```python
from build123d import *

# Parameters (mm, degrees)
F1_DEPTH     = 12
F2_T1_DEPTH  = 40.9442549995
F2_T3_DEPTH  = 65.4442549995
F2_T5_DEPTH  = 40.9442549995
F2_T7_DEPTH  = 10.4442549995
F2_T9_DEPTH  = 10.4442549995
F2_T12_ANGLE = 68.042658845
F3_W         = 6
F3_H         = 5
F4_DEPTH     = 50.251
F8_DEPTH     = 70.251
F10_DEPTH    = 3


# Not quite as in the source:
# - a fillet or chamfer that OpenCascade refuses, or shapes differently, is made with other operations: its cross-section is extruded or revolved along the edge and cut away or added


with BuildPart() as f1:
    # F0 (on Top) → F1 (new body)
    with BuildSketch(Plane.XY):
        with BuildLine():
            Line((-35.125, 35.3986228546), (-30.125, 0))
            Line((-30.125, 0), (0, 0))
            Line((0, 0), (0, 1.25))
            Line((0, 1.25), (-29.0391526732, 1.25))
            Line((-29.0391526732, 1.25), (-33.8579983297, 35.3660999978))
            Line((-33.8579983297, 35.3660999978), (-33.0027387168, 39.7740071493))
            ThreePointArc((-33.0027387168, 39.7740071493), (-17.1340283274, 46.6501181236), (0, 49))
            Line((0, 49), (0, 50.25))
            ThreePointArc((0, 50.25), (-17.738073715, 47.7785625378), (-34.125, 40.5525048866))
            Line((-34.125, 40.5525048866), (-35.125, 35.3986228546))
        make_face()
        with BuildLine():
            Line((0, 1.25), (0, 0))
            Line((0, 0), (30.125, 0))
            Line((30.125, 0), (35.125, 35.3986228546))
            Line((35.125, 35.3986228546), (34.125, 40.5525048866))
            ThreePointArc((34.125, 40.5525048866), (17.738073715, 47.7785625378), (0, 50.25))
            Line((0, 50.25), (0, 49))
            ThreePointArc((0, 49), (17.1340283274, 46.6501181236), (33.0027387168, 39.7740071493))
            Line((33.0027387168, 39.7740071493), (33.8579983297, 35.3660999978))
            Line((33.8579983297, 35.3660999978), (29.0391526732, 1.25))
            Line((29.0391526732, 1.25), (0, 1.25))
        make_face()
    extrude(amount=F1_DEPTH)

    # F2: chamfer of 0.25 x 1 on 6 edges, made by hand

    # F2_s2 → F2_t1 (cut)
    with BuildSketch(Plane(origin=(-5.9525054843, 42.142099336, 0), x_dir=(0, 0, 1), z_dir=(0.1398601399, -0.9901712687, 0))):
        Polygon((11, 29.8289094684), (12, 29.5789094684), (12, 29.8289094684), align=None)
    extrude(amount=F2_T1_DEPTH, mode=Mode.SUBTRACT)

    # F2_s4 → F2_t3 (cut)
    with BuildSketch(Plane.YZ.offset(-32.7221274998)):
        Polygon((0, 11), (0.25, 12), (0, 12), align=None)
    extrude(amount=F2_T3_DEPTH, mode=Mode.SUBTRACT)

    # F2_s6 → F2_t5 (cut)
    with BuildSketch(Plane(origin=(0.2260362536, 1.6002744188, 0), x_dir=(0, 0, 1), z_dir=(0.1398601399, 0.9901712687, 0))):
        Polygon((11, 29.8289094684), (12, 29.5789094684), (12, 29.8289094684), align=None)
    extrude(amount=F2_T5_DEPTH, mode=Mode.SUBTRACT)

    # F2_s8 → F2_t7 (cut)
    with BuildSketch(Plane(origin=(-4.8500827906, 24.9967545481, 0), x_dir=(0, 0, 1), z_dir=(-0.1904761905, 0.9816918156, 0))):
        Polygon((11, 41.2245198532), (12, 40.9745198532), (12, 41.2245198532), align=None)
    extrude(amount=F2_T7_DEPTH, mode=Mode.SUBTRACT)

    # F2_s10 → F2_t9 (cut)
    with BuildSketch(Plane(origin=(6.8394646952, 35.2497942014, 0), x_dir=(0, 0, 1), z_dir=(-0.1904761905, -0.9816918156, 0))):
        Polygon((11, 41.2245198532), (12, 40.9745198532), (12, 41.2245198532), align=None)
    extrude(amount=F2_T9_DEPTH, mode=Mode.SUBTRACT)

    # F2_s11 → F2_t12 (revolve, cut)
    with BuildSketch(Plane(origin=(6.7894109874, -4.5831938529, 0), x_dir=(0, 0, 1), z_dir=(0.8288293451, -0.5595014894, 0))):
        Polygon((11, -52.7560806603), (12, -52.5060806603), (12, -52.7560806603), align=None)
    revolve(axis=Axis((0, -14.6408311763, 12), (0, 0, 1)), revolution_arc=F2_T12_ANGLE, mode=Mode.SUBTRACT)

    # F3 (on face) → F4 (cut, through all)
    with BuildSketch(Plane.XZ):
        with Locations((-18.4078305346, 8.5)):
            Rectangle(F3_W, F3_H)
        Polygon((-21.9078305346, 12), (-21.4078305346, 11), (-15.4078305346, 11), (-14.9078305346, 12), align=None)
        with Locations((18.4078305346, 8.5)):
            Rectangle(F3_W, F3_H)
        Polygon((14.9078305346, 12), (15.4078305346, 11), (21.4078305346, 11), (21.9078305346, 12), align=None)
        with Locations((-5.25, 4.5)):
            Rectangle(F3_W, F3_H)
        with Locations((5.25, 4.5)):
            Rectangle(F3_W, F3_H)
    extrude(amount=-F4_DEPTH, mode=Mode.SUBTRACT)

    # F7 (on face) → F8 (cut, through all)
    with BuildSketch(Plane(origin=(-35.125, 0, 0), x_dir=(0, -1, 0), z_dir=(-1, 0, 0))):
        Polygon((-19.0282890696, 12), (-18.5332034352, 11), (-18.5332034352, 6), (-12.5921758233, 6), (-12.5921758233, 11), (-12.0970901889, 12), align=None)
    extrude(amount=-F8_DEPTH, mode=Mode.SUBTRACT)

    # F9 (on face) + F0 (on Top) → F10 (join)
    with BuildSketch(Plane(origin=(0, 0, 0), x_dir=(1, 0, 0), z_dir=(0, 0, -1))):
        with BuildLine():
            Line((30.125, 0), (-30.125, 0))
            Line((-30.125, 0), (-35.125, -35.3986228546))
            Line((-35.125, -35.3986228546), (-34.125, -40.5525048866))
            ThreePointArc((-34.125, -40.5525048866), (0, -50.25), (34.125, -40.5525048866))
            Line((34.125, -40.5525048866), (35.125, -35.3986228546))
            Line((35.125, -35.3986228546), (30.125, 0))
        make_face()
        with BuildLine():
            Line((-33.8579983297, -35.3660999978), (-29.0391526732, -1.25))
            Line((-29.0391526732, -1.25), (29.0391526732, -1.25))
            Line((29.0391526732, -1.25), (33.8579983297, -35.3660999978))
            Line((33.8579983297, -35.3660999978), (33.0027387168, -39.7740071493))
            ThreePointArc((33.0027387168, -39.7740071493), (0, -49), (-33.0027387168, -39.7740071493))
            Line((-33.0027387168, -39.7740071493), (-33.8579983297, -35.3660999978))
        make_face(mode=Mode.SUBTRACT)
    with BuildSketch(Plane.XY):
        with BuildLine():
            Line((-35.125, 35.3986228546), (-30.125, 0))
            Line((-30.125, 0), (0, 0))
            Line((0, 0), (0, 1.25))
            Line((0, 1.25), (-29.0391526732, 1.25))
            Line((-29.0391526732, 1.25), (-33.8579983297, 35.3660999978))
            Line((-33.8579983297, 35.3660999978), (-33.0027387168, 39.7740071493))
            ThreePointArc((-33.0027387168, 39.7740071493), (-17.1340283274, 46.6501181236), (0, 49))
            Line((0, 49), (0, 50.25))
            ThreePointArc((0, 50.25), (-17.738073715, 47.7785625378), (-34.125, 40.5525048866))
            Line((-34.125, 40.5525048866), (-35.125, 35.3986228546))
        make_face()
        with BuildLine():
            Line((0, 1.25), (0, 0))
            Line((0, 0), (30.125, 0))
            Line((30.125, 0), (35.125, 35.3986228546))
            Line((35.125, 35.3986228546), (34.125, 40.5525048866))
            ThreePointArc((34.125, 40.5525048866), (17.738073715, 47.7785625378), (0, 50.25))
            Line((0, 50.25), (0, 49))
            ThreePointArc((0, 49), (17.1340283274, 46.6501181236), (33.0027387168, 39.7740071493))
            Line((33.0027387168, 39.7740071493), (33.8579983297, 35.3660999978))
            Line((33.8579983297, 35.3660999978), (29.0391526732, 1.25))
            Line((29.0391526732, 1.25), (0, 1.25))
        make_face()
    extrude(amount=F10_DEPTH, dir=(0, 0, -1))


solid = f1.part
```
Check sheet for the modelled part. Datum: model origin and axes. Units: mm. A direction names the side the tool comes from. Coordinates: 2 decimals unless noted, no trailing zeros. Order: outer loops, then holes, each group sorted by start corner. A loop starts at its lowest first (then second) coordinate and runs counter-clockwise, first axis right, second up. Notation, with made-up numbers: M 42.25,73 L 75.25,73 A14 ccw 75.25,99 Z; hole C 8,42 d4. An arc over 180 degrees is marked long. Write each question's results on one line, items separated by ' | '. Start each with the question number.
1. Material ranges on probe 1 along Y at (x, z) = (-0.5, 2); probe 2 along X at (y, z) = (28, 5.75); probe 3 along X at (y, z) = (42.5, 8), recorded low to high.
2. Cross-section at D-D on y = 24. Record the cut outline in (x, z), and give its area (3 significant figures).
3. Access from +Z, -Z, +X, -X, +Y, -Y to the whole of each face (thin tool, end or side, straight path). Record for faces 4 (the face through (-18, 47, 6)), 5 (the face through (-5, 49, 7)), 6 (the face through (-32, 16, 6)), 7 (the face through (31.415, 18.069, 4.605)).
4. Mould release check, pull along Z, two halves, no side actions. Record for faces 1 (the face through (5, 49, 2)), 2 (the face through (21.408, 46, 8)), 3 (the face through (0.2, 50.1, 11.6)): +Z half, -Z half, draft (parallel to the pull), parting line (faces both ways), or undercut.
5. Cross-section at B-B on x = -20.5. Record the cut outline in (y, z), and give its area (3 significant figures).
6. Cross-section at A-A on z = 3.25. State how many separate pieces and enclosed holes the cut face has, and give its area (3 significant figures).
7. Go/stop test with flat-tipped pins: P1, Ø1.7, axis at x = -31, y = 16, coming from the +Z side; P2, Ø0.6, axis at y = 47.5, z = 8.5, coming from the -X side; P3, Ø1.5, axis at y = 23.5, z = 3.5, coming from the -X side; P4, Ø8, axis at x = -22.5, y = 40, coming from the -Z side. Record where each tip stops, or that it passes through.
Checks:
1) probe 1: y = 0 to 1.25, 49 to 50.25 | probe 2: x = -34.08 to -32.82, 32.82 to 34.08 | probe 3: x = -30.75 to -28.02, 28.02 to 30.75
2) outline: M -33.51,-3 L -32.25,-3 L -32.25,12 L -33.26,12 L -33.51,11 Z; M 32.25,-3 L 33.51,-3 L 33.51,11 L 33.26,12 L 32.25,12 Z | area: 37.6 mm²
3) face 4: +Z, +Y, -Y | face 5: +Y, -Y | face 6: +Z, +X, -X | face 7: +Z, -Z
4) face 1: undercut | face 2: draft | face 3: +Z half
5) outline: M 0,-3 L 1.25,-3 L 1.25,6 L 0,6 Z; M 45.61,-3 L 46.93,-3 L 46.93,6 L 45.61,6 Z | area: 23.1 mm²
6) separate pieces: 4 | enclosed holes: 0 | area: 232 mm²
7) P1: stops at z = 6 | P2: stops at x = -15.41 | P3: stops at x = -33.55 | P4: passes through
